Build history of the part. All positions in model axes, mm. Give positions to 0.01 mm unless a question says otherwise; leave off trailing zeros. Order: outer loops, then holes, each group sorted by start corner. A loop starts at its lowest first (then second) coordinate and runs counter-clockwise, first axis right, second up. Notation, with made-up numbers: (-37.5, 46.5) - (17.5, 46.5) arc R23 cw to (17.5, 62.5) - close; hole circle Ø3 at (73.5, -27.5). An arc over 180 degrees is marked (long way). Write each question's results on one line, items separated by ' | '. Start each with the question number.
1) Drop a flat-ended pin along its axis: pin 1 Ø3 at (x, y) = (-40, -48) entering from -Z. Give the stop position or say it passes through.
2) Cut at A-A on y = -48. List the corners of the cut face in (x, z).
3) Drill centre lines: line 1 along Y through (x, z) = (-40, 2.4); line 2 along X through (y, z) = (-56.5, 2.7); line 3 along X through (y, z) = (52.5, 0.55). Where is each one in solid material? Low to high. Write a range as from..to.
4) Cut at C-C on z = 2.45. State how many separate pieces and enclosed holes the cut face has, plus the area to 3 significant figures.
5) Two-plate mould, pull along Y, no slides. Class faces 1 (the face through (44.108, -53.101, 1.479)), 2 (the face through (-1, 1, 0)): +Y half, -Y half, draft (parallel to the pull), parting line (faces both ways), or undercut.
from build123d import *

# Parameters (mm, degrees)
F0_W     = 128
F0_H     = 128
F0_R     = 1.85
F0_R_2   = 4
F1_DEPTH = 3


with BuildPart() as f1:
    # F0 (on Top) → F1 (new body)
    with BuildSketch(Plane.XY):
        Rectangle(F0_W, F0_H)
        with Locations((-53.656854, -53.656854)):
            Circle(F0_R, mode=Mode.SUBTRACT)
        with Locations((-48, -56)):
            Circle(F0_R, mode=Mode.SUBTRACT)
        with Locations((-42.343146, -53.656854)):
            Circle(F0_R, mode=Mode.SUBTRACT)
        with Locations((-56, -48)):
            Circle(F0_R, mode=Mode.SUBTRACT)
        with Locations((-53.656854, -42.343146)):
            Circle(F0_R, mode=Mode.SUBTRACT)
        with Locations((-48, -48)):
            Circle(F0_R_2, mode=Mode.SUBTRACT)
        with Locations((-42.343146, -42.343146)):
            Circle(F0_R, mode=Mode.SUBTRACT)
        with Locations((-40, -48)):
            Circle(F0_R, mode=Mode.SUBTRACT)
        with Locations((-48, -40)):
            Circle(F0_R, mode=Mode.SUBTRACT)
        with Locations((42.343146, -53.656854)):
            Circle(F0_R, mode=Mode.SUBTRACT)
        with Locations((48, -56)):
            Circle(F0_R, mode=Mode.SUBTRACT)
        with Locations((53.656854, -53.656854)):
            Circle(F0_R, mode=Mode.SUBTRACT)
        with Locations((40, -48)):
            Circle(F0_R, mode=Mode.SUBTRACT)
        with Locations((42.343146, -42.343146)):
            Circle(F0_R, mode=Mode.SUBTRACT)
        with Locations((48, -48)):
            Circle(F0_R_2, mode=Mode.SUBTRACT)
        with Locations((53.656854, -42.343146)):
            Circle(F0_R, mode=Mode.SUBTRACT)
        with Locations((56, -48)):
            Circle(F0_R, mode=Mode.SUBTRACT)
        with Locations((48, -40)):
            Circle(F0_R, mode=Mode.SUBTRACT)
        with Locations((-53.656854, 42.343146)):
            Circle(F0_R, mode=Mode.SUBTRACT)
        with Locations((-48, 40)):
            Circle(F0_R, mode=Mode.SUBTRACT)
        with Locations((-42.343146, 42.343146)):
            Circle(F0_R, mode=Mode.SUBTRACT)
        with Locations((-56, 48)):
            Circle(F0_R, mode=Mode.SUBTRACT)
        with Locations((-53.656854, 53.656854)):
            Circle(F0_R, mode=Mode.SUBTRACT)
        with Locations((-48, 48)):
            Circle(F0_R_2, mode=Mode.SUBTRACT)
        with Locations((-42.343146, 53.656854)):
            Circle(F0_R, mode=Mode.SUBTRACT)
        with Locations((-40, 48)):
            Circle(F0_R, mode=Mode.SUBTRACT)
        with Locations((-48, 56)):
            Circle(F0_R, mode=Mode.SUBTRACT)
        with Locations((42.343146, 42.343146)):
            Circle(F0_R, mode=Mode.SUBTRACT)
        with Locations((48, 40)):
            Circle(F0_R, mode=Mode.SUBTRACT)
        with Locations((53.656854, 42.343146)):
            Circle(F0_R, mode=Mode.SUBTRACT)
        with Locations((40, 48)):
            Circle(F0_R, mode=Mode.SUBTRACT)
        with Locations((42.343146, 53.656854)):
            Circle(F0_R, mode=Mode.SUBTRACT)
        with Locations((48, 48)):
            Circle(F0_R_2, mode=Mode.SUBTRACT)
        with Locations((53.656854, 53.656854)):
            Circle(F0_R, mode=Mode.SUBTRACT)
        with Locations((56, 48)):
            Circle(F0_R, mode=Mode.SUBTRACT)
        with Locations((48, 56)):
            Circle(F0_R, mode=Mode.SUBTRACT)
    extrude(amount=F1_DEPTH)


solid = f1.part
Results:
1) pin 1: through
2) outline: (-64, 0) - (-57.85, 0) - (-57.85, 3) - (-64, 3) - close; (-54.15, 0) - (-52, 0) - (-52, 3) - (-54.15, 3) - close; (-44, 0) - (-41.85, 0) - (-41.85, 3) - (-44, 3) - close; (-38.15, 0) - (38.15, 0) - (38.15, 3) - (-38.15, 3) - close; (41.85, 0) - (44, 0) - (44, 3) - (41.85, 3) - close; (52, 0) - (54.15, 0) - (54.15, 3) - (52, 3) - close; (57.85, 0) - (64, 0) - (64, 3) - (57.85, 3) - close
3) line 1: -64..-49.85, -46.15..46.15, 49.85..64 | line 2: -64..-49.78, -46.22..46.22, 49.78..64 | line 3: -64..-55.1, -52.21..-43.79, -40.9..40.9, 43.79..52.21, 55.1..64
4) separate pieces: 1 | enclosed holes: 36 | area: 15,800 mm^2
5) face 1: undercut | face 2: draft
